from build123d import *

# Parameters (mm, degrees)
BOSS_EXTRUDE1_DEPTH = 21
SHELL1_T            = -1.6
SKETCH2_R           = 6.8
CUT_EXTRUDE1_DEPTH  = 2


with BuildPart() as part:
    # Sketch1 → Boss-Extrude1 (new, symmetric)
    with BuildSketch(Plane(origin=(0, 0, 0), x_dir=(0, 0, -1), z_dir=(1, 0, 0))):
        Polygon((-34.96784237, -1.5), (34.96784237, 1.5), (34.96784237, 6.5), (-34.96784237, 6.5), align=None)
    extrude(amount=BOSS_EXTRUDE1_DEPTH, both=True)

    # Shell1
    shell1_openings = [part.faces().sort_by_distance(p)[0] for p in [
        (0, 6.5, 0),
    ]]
    offset(amount=SHELL1_T, openings=shell1_openings, kind=Kind.INTERSECTION)

    # Sketch2 → Cut-Extrude1 (cut)
    with BuildSketch(Plane.XY.offset(34.96784237)):
        with Locations((0, 6.5)):
            Circle(SKETCH2_R)
    extrude(amount=-CUT_EXTRUDE1_DEPTH, mode=Mode.SUBTRACT)


solid = part.part
Work out the finished part from the listing and answer in its coordinate system (mm). A direction names the side the tool comes from. Round coordinates to 2 decimals unless told otherwise and drop trailing zeros. Loops run counter-clockwise (first coordinate to the right, second up) from the corner with the lowest first, then second, coordinate; pieces in that order, holes last. Notation, with made-up numbers: (-27.5, 34.5) - (-13.5, 34.5) arc R22 ccw to (-13.5, 45.5) - close; hole circle Ø6 at (-15.75, 55). An arc over 180 degrees is marked (long way). One line per item, written item: value.
Q1. Straight lines are drawn through the part: probe 1 along X at (y, z) = (3.25, 15); probe 2 along Z at (x, y) = (-9.5, 5); probe 3 along Z at (x, y) = (0, 5.5). For each, find the intervals that lie inside material, in ascending order.
Check values:
probe 1: -21 to -19.4, 19.4 to 21
probe 2: -34.97 to -33.37, 33.37 to 34.97
probe 3: -34.97 to -33.37
Q2. Find section B-B on y = 5.75. Give the vertices of the cut face in (x, z), and give its area (3 significant figures).
Check values:
outline: (-21, -34.97) - (21, -34.97) - (21, 34.97) - (6.76, 34.97) - (6.76, 33.37) - (19.4, 33.37) - (19.4, -33.37) - (-19.4, -33.37) - (-19.4, 33.37) - (-6.76, 33.37) - (-6.76, 34.97) - (-21, 34.97) - close
area: 326 mm2
Q3. Each of these flat-tipped pins is pushed along its axis until it touches: pin 1 Ø4 at (x, z) = (-15, 1.5) entering from +Y; pin 2 Ø8 at (x, z) = (12.5, 19) entering from -Y; pin 3 Ø1.5 at (x, z) = (6, -5) entering from +Y. Where does it stop, or does it pass through?
Check values:
pin 1: y = 1.62
pin 2: y = -0.99
pin 3: y = 1.85
Q4. Find section A-A on x = -17. Give the vertices of the cut face in (y, z).
Check values:
outline: (-1.5, 34.97) - (1.5, -34.97) - (6.5, -34.97) - (6.5, -33.37) - (3.03, -33.37) - (0.17, 33.37) - (6.5, 33.37) - (6.5, 34.97) - close
Q5. The mould has two halves that part along Z. Classify faces 4 (the flat face through (0, 4, -34.968)), 5 (the flat face through (-19.4, 4, 0)), 6 (the flat face through (21, 3, 0)): +Z half, -Z half, draft (parallel to the pull), parting line (faces both ways), or undercut.
Check values:
face 4: -Z half
face 5: undercut
face 6: draft
Q6. For faces 1 (the flat face through (0, 0, 0)), 2 (the cylindrical face through (-0.1, -0.3, 34.2)), 3 (the flat face through (0.27, 1.58, 0.47)), determine the directions among +Z, -Z, +X, -X, +Y, -Y from which every point of the face is accessible in a straight line to the end or side of a thin tool.
Check values:
face 1: -Z, +X, -X, -Y
face 2: +Z, +Y
face 3: +Y
Q7. Find section C-C on z = 21.5. Give the vertices of the cut face in (x, y), and give its area (3 significant figures).
Check values:
outline: (-21, -0.92) - (21, -0.92) - (21, 6.5) - (19.4, 6.5) - (19.4, 0.68) - (-19.4, 0.68) - (-19.4, 6.5) - (-21, 6.5) - close
area: 85.9 mm2
